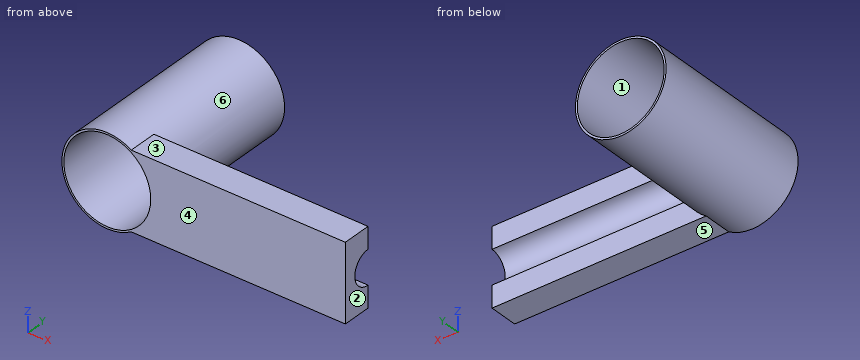
Autodesk Inventor part; units mm, degrees
ref_plane "YZ Plane" through (0, 0, 0) normal (1, 0, 0) x (0, 1, 0)
ref_plane "XZ Plane" through (0, 0, 0) normal (0, 1, 0) x (-1, 0, 0)
ref_plane "XY Plane" through (0, 0, 0) normal (0, 0, 1) x (1, 0, 0)
sketch "草圖1" plane through (0, 0, 0) normal (1, 0, 0) x (0, 1, 0)
  arc A0 (0, 17.5) -> (0, -17.5) centre (0, 0) ccw
  arc A1 (0, 20) -> (0, -20) centre (0, 0) ccw
  line L0 (0, 17.5) -> (0, 20)
  line L1 (0, -20) -> (0, -17.5)
  line L2 (0, -56) -> (0, 56)
  line L3 (0, -40) -> (-30, -40)
  line L4 (-30, -40) -> (-30, -20)
  line L5 (0, -40) -> (0, -20)
  line L6 (-36, 0) -> (6, 0)
  line L7 (0, 40) -> (-30, 40)
  line L8 (-30, 40) -> (-30, -20)
  point P0 (0, -20)
  dimension "d0" = 17.5
  dimension "d1" = 20
  dimension "d4" = 30
  dimension "d5" = 40
extrude "擠出1" add sketch "草圖1" along normal blind 200 contours A0 L6 A1 L0 | A0 L1 A1 L6 | A1 L6 L8 L7 L2 | A1 L2 L3 L4 L8 L6
sketch "草圖3" plane through (0, -30, -40) normal (0, -1, 0) x (1, 0, 0)
  circle A0 centre (-47.101, 40) radius 45.101
  circle A1 centre (-47.101, 40) radius 47.101
  line L0 (-153.0424, 40) -> (258.8404, 40)
  line L1 (0, 80) -> (0, 0)
  point P0 (0, 40)
  dimension "d6" = 90.202
  dimension "d7" = 2
extrude "擠出2" add sketch "草圖3" against normal blind 175 contours L0 A1 A0 | A0 L0 A1
extrude "擠出3" add sketch "草圖1" against normal up to surface contours A0 L6 A1 L0 | A0 L1 A1 L6 | A1 L6 L8 L7 L2 | A1 L2 L3 L4 L8 L6
sketch "草圖4" plane through (200, 0, 0) normal (1, 0, 0) x (0, 0, -1)
  arc A0 (-17.5, 0) -> (17.5, 0) centre (0, 0) ccw
  circle A1 centre (0, 0) radius 17.5
extrude "擠出4" cut sketch "草圖4" against normal up to surface
properties part number "直線軌道"
Could you check a few things on this model? Use its own coordinates, in mm. Face numbers are marked on the shaded views. A direction names the side the tool comes from. Round coordinates to 2 decimals unless told otherwise and drop trailing zeros. Loops run counter-clockwise (first coordinate to the right, second up) from the corner with the lowest first, then second, coordinate; pieces in that order, holes last. Notation, with made-up numbers: (58.25, 51) -> (108.25, 51) arc R38 ccw to (108.25, 90) -> close; hole circle Ø8 at (-36, 31). An arc over 180 degrees is marked (long way). Put each result on its own line as item: value.
Q1. Which directions (+Z, -Z, +X, -X, +Y, -Y) give clear straight access to the entire face, cutting with the end or side of a thin tool? Please do the marked faces 4, 5 and 6.
Checks:
face 4: +Z, -Z, +X, -X, -Y
face 5: -Z, +X, +Y, -Y
face 6: +Y
Q2. I want a section at D-D on y = 130. Write out the boundary of the cut face in (x, z).
Checks:
outline: circle Ø94.2 at (-47.1, 0); hole circle Ø90.2 at (-47.1, 0)
Q3. I want a section at A-A on z = 0. Write out the boundary of the cut face in (x, y), and give its area (3 significant figures).
Checks:
outline: (-94.2, -30) -> (-92.2, -30) -> (-92.2, 145) -> (-94.2, 145) -> close; (-2, -30) -> (200, -30) -> (200, -17.5) -> (-2, -17.5) -> close; (-2, 17.5) -> (0, 17.5) -> (0, 145) -> (-2, 145) -> close
area: 3,130 mm2
Q4. For pin 1 Ø12 at (x, z) = (6.5, 26) entering from +Y; pin 2 Ø9 at (x, y) = (103.5, -11) entering from +Z; pin 3 Ø8 at (y, z) = (57.5, -33.5) entering from +X, each with a flat end and sliding along its axis, tell me the tip position at first contact or that it passes through.
Checks:
pin 1: y = 0
pin 2: z = 40
pin 3: x = -10.38
Q5. I want a section at B-B on x = -74. Write out the boundary of the cut face in (y, z).
Checks:
outline: (-30, -38.66) -> (145, -38.66) -> (145, -36.2) -> (-30, -36.2) -> close; (-30, 36.2) -> (145, 36.2) -> (145, 38.66) -> (-30, 38.66) -> close
Q6. Please list where these lines run through material, in increasing order: line 1 (Y direction, x = 129.5, z = 0); line 2 (Z direction, x = 135, y = -9); line 3 (X direction, y = 49.5, z = 13). Write a range as from..to.
Checks:
line 1: -30..-17.5
line 2: -40..-15.01, 15.01..40
line 3: -92.37..-90.29, -3.91..-1.83
Q7. I want a section at C-C on z = 33. Write out the boundary of the cut face in (x, y), and give its area (3 significant figures).
Checks:
outline: (-80.71, -30) -> (-77.84, -30) -> (-77.84, 145) -> (-80.71, 145) -> close; (-16.36, -30) -> (200, -30) -> (200, 0) -> (-13.49, 0) -> (-13.49, 145) -> (-16.36, 145) -> close
area: 7,410 mm2
Q8. Thinking about a two-plate mould opening in X: for the marked faces 1, 2 and 3, which applies, pulls with the +X half, pulls with the -X half, needs draft (parallel to the pull), parting line crosses it, or undercut?
Checks:
face 1: undercut
face 2: pulls with the +X half
face 3: needs draft
